from build123d import *

# Parameters (mm, degrees)
SKETCH1_W           = 65
SKETCH1_H           = 46
SKETCH1_R           = 1.5
BOSS_EXTRUDE1_DEPTH = 5
SKETCH2_R           = 2
CUT_EXTRUDE1_DEPTH  = 10
SKETCH3_W           = 4
SKETCH3_H           = 46
CUT_EXTRUDE2_DEPTH  = 6
SKETCH4_W           = 6
SKETCH4_H           = 46
BOSS_EXTRUDE2_DEPTH = 5
FILLET1_R           = 10
FILLET2_R           = 1
SKETCH2_3_R         = 2
CUT_EXTRUDE3_DEPTH  = 10


with BuildPart() as part:
    # Sketch1 → Boss-Extrude1 (new body)
    with BuildSketch(Plane.XY):
        with Locations((7.5, 0)):
            Rectangle(SKETCH1_W, SKETCH1_H)
        with BuildLine():
            ThreePointArc((4.6, 0), (3.252691193, -3.252691193), (0, -4.6))
            ThreePointArc((0, -4.6), (-3.252691193, 3.252691193), (4.6, 0))
        make_face(mode=Mode.SUBTRACT)
        with Locations((30, -18.25)):
            Circle(SKETCH1_R, mode=Mode.SUBTRACT)
        with BuildLine():
            ThreePointArc((1.5, -10), (-1.060660172, -11.060660172), (0, -8.5))
            ThreePointArc((0, -8.5), (1.060660172, -8.939339828), (1.5, -10))
        make_face(mode=Mode.SUBTRACT)
        with BuildLine():
            ThreePointArc((39.5, 0), (23.282485579, -6.717514421), (30, 9.5))
            ThreePointArc((30, 9.5), (36.717514421, 6.717514421), (39.5, 0))
        make_face(mode=Mode.SUBTRACT)
        with Locations((0, 10)):
            Circle(SKETCH1_R, mode=Mode.SUBTRACT)
        with BuildLine():
            ThreePointArc((31.5, 18.25), (31.060660172, 17.189339828), (30, 16.75))
            ThreePointArc((30, 16.75), (28.939339828, 19.310660172), (31.5, 18.25))
        make_face(mode=Mode.SUBTRACT)
    extrude(amount=BOSS_EXTRUDE1_DEPTH)

    # Sketch2 → Cut-Extrude1 (cut)
    with BuildSketch(Plane.XY.offset(5)):
        with Locations((7, 19)):
            Circle(SKETCH2_R)
        with Locations((-5, -19)):
            Circle(SKETCH2_R)
        with Locations((-17, 19)):
            Circle(SKETCH2_R)
        with Locations((-5, 19)):
            Circle(SKETCH2_R)
        with Locations((7, -19)):
            Circle(SKETCH2_R)
        with Locations((-17, -19)):
            Circle(SKETCH2_R)
    extrude(amount=-CUT_EXTRUDE1_DEPTH, mode=Mode.SUBTRACT)

    # Sketch3 → Cut-Extrude2 (cut, through all)
    with BuildSketch(Plane.XY.offset(5)):
        with Locations((-23, 0)):
            Rectangle(SKETCH3_W, SKETCH3_H)
    extrude(amount=-CUT_EXTRUDE2_DEPTH, mode=Mode.SUBTRACT)

    # Sketch4 → Boss-Extrude2 (add)
    with BuildSketch(Plane.XY.offset(5)):
        with Locations((43, 0)):
            Rectangle(SKETCH4_W, SKETCH4_H)
    extrude(amount=-BOSS_EXTRUDE2_DEPTH)

    # Fillet1
    fillet1_edges = [part.edges().sort_by_distance(p)[0] for p in [
        (46, -23, 2.5),
        (46, 23, 2.5),
    ]]
    fillet(fillet1_edges, radius=FILLET1_R)

    # Fillet2
    fillet2_edges = [part.edges().sort_by_distance(p)[0] for p in [
        (-21, 23, 2.5),
        (-21, -23, 2.5),
    ]]
    fillet(fillet2_edges, radius=FILLET2_R)

    # Sketch2<3> → Cut-Extrude3 (cut)
    with BuildSketch(Plane.XY.offset(5)):
        with Locations((19, -19)):
            Circle(SKETCH2_3_R)
    extrude(amount=-CUT_EXTRUDE3_DEPTH, mode=Mode.SUBTRACT)


solid = part.part
The model under review builds one solid part; all positions refer to its coordinate system, in mm. Give positions to 0.01 mm unless a question says otherwise; leave off trailing zeros. Write each loop counter-clockwise with the first axis right and the second up, starting at its lowest first coordinate (ties: lowest second). Pieces come first, ordered by that corner, then holes.
1. Add section B-B, the plane y = -18.25. Write out the cut boundary in (x, z), plus the area to 3 significant figures.
2. Add section D-D, the plane y = 19. Write out the cut boundary in (x, z), plus the area to 3 significant figures.
3. For P1, Ø2.5, axis at x = 7, y = -19, coming from the +Z side, flat-tipped, find the tip position at first contact; note if it passes through.
4. Draft analysis for pull direction X (two halves, no side actions). For faces 1 (the cylindrical face through (28.5, -18.2, 2.5)), 2 (the cylindrical face through (-0.325, 8.536, 2.465)), 3 (the flat face through (-21, 0, 3)), 4 (the flat face through (46, 0, 3)), state which applies: +X half, -X half, draft (parallel to the pull), parting line (faces both ways), or undercut.
5. Add section C-C, the plane z = 4.25. Count the separate pieces of the cut face and the enclosed holes in it, plus the area to 3 significant figures.
6. Wall thickness on L1, parallel to Y at x = -17, z = 2.25; L2, parallel to Y at x = 30, z = 1; L3, parallel to Y at x = -16.5, z = 4.1: over which ranges is each line inside the solid? List them lowest first.
7. Add section A-A, the plane x = 19. Write out the cut boundary in (y, z), plus the area to 3 significant figures.
Worked answers:
1. outline: (-21, 0) - (-18.85, 0) - (-18.85, 5) - (-21, 5) - close; (-15.15, 0) - (-6.85, 0) - (-6.85, 5) - (-15.15, 5) - close; (-3.15, 0) - (5.15, 0) - (5.15, 5) - (-3.15, 5) - close; (8.85, 0) - (17.15, 0) - (17.15, 5) - (8.85, 5) - close; (20.85, 0) - (28.5, 0) - (28.5, 5) - (20.85, 5) - close; (31.5, 0) - (44.51, 0) - (44.51, 5) - (31.5, 5) - close
1. area: 238 mm2
2. outline: (-21, 0) - (-19, 0) - (-19, 5) - (-21, 5) - close; (-15, 0) - (-7, 0) - (-7, 5) - (-15, 5) - close; (-3, 0) - (5, 0) - (5, 5) - (-3, 5) - close; (9, 0) - (28.7, 0) - (28.7, 5) - (9, 5) - close; (31.3, 0) - (44, 0) - (44, 5) - (31.3, 5) - close
2. area: 252 mm2
3. P1: passes through
4. face 1: undercut
4. face 2: undercut
4. face 3: -X half
4. face 4: +X half
5. separate pieces: 1
5. enclosed holes: 13
5. area: 2,570 mm2
6. L1: y = -23 to -21, -17 to 17, 21 to 23
6. L2: y = -23 to -19.75, -16.75 to -9.5, 9.5 to 16.75, 19.75 to 23
6. L3: y = -23 to -20.94, -17.06 to 17.06, 20.94 to 23
7. outline: (-23, 0) - (-21, 0) - (-21, 5) - (-23, 5) - close; (-17, 0) - (23, 0) - (23, 5) - (-17, 5) - close
7. area: 210 mm2
